For this review, take the finished solid that the model builds, in its own axes (mm). Give positions to 0.01 mm unless a question says otherwise; leave off trailing zeros. Loops run counter-clockwise (first coordinate to the right, second up) from the corner with the lowest first, then second, coordinate; pieces in that order, holes last.
```python
from build123d import *

# Parameters (mm, degrees)
ESQUISSE1_R             = 57.75
BOSS_EXTRU_1_DEPTH      = 1
ESQUISSE2_R             = 4
ENL_V_MAT_EXTRU_1_DEPTH = 10
ENL_V_MAT_EXTRU_4_DEPTH = 10
ESQUISSE5_R             = 1.5
ENL_V_MAT_EXTRU_5_DEPTH = 10


with BuildPart() as part:
    # Esquisse1 → Boss.-Extru.1 (new body)
    with BuildSketch(Plane.XY):
        Circle(ESQUISSE1_R)
    extrude(amount=BOSS_EXTRU_1_DEPTH)

    # Esquisse2 → Enlèv. mat.-Extru.1 (cut)
    with BuildSketch(Plane.XY.offset(1)):
        Circle(ESQUISSE2_R)
    extrude(amount=-ENL_V_MAT_EXTRU_1_DEPTH, mode=Mode.SUBTRACT)

    # Esquisse4 → Enlèv. mat.-Extru.4 (cut)
    with BuildSketch(Plane(origin=(0, 0, 0), x_dir=(-1, 0, 0), z_dir=(0, 0, -1))):
        with BuildLine():
            Line((33.243703386, 10.947884963), (53.229228234, 18.16877802))
            ThreePointArc((53.229228234, 18.16877802), (55.31077904, 10.615789501), (56.184630477, 2.830105651))
            Line((56.184630477, 2.830105651), (34.934630477, 2.138128484))
            ThreePointArc((34.934630477, 2.138128484), (34.372579979, 6.597404459), (33.243703386, 10.947884963))
        make_face()
    extrude(amount=-ENL_V_MAT_EXTRU_4_DEPTH, mode=Mode.SUBTRACT)

    # Esquisse5 → Enlèv. mat.-Extru.5 (cut)
    with BuildSketch(Plane(origin=(0, 0, 0), x_dir=(-1, 0, 0), z_dir=(0, 0, -1))):
        with Locations((0.504599234, -15.495791231)):
            Circle(ESQUISSE5_R)
    extrude(amount=-ENL_V_MAT_EXTRU_5_DEPTH, mode=Mode.SUBTRACT)


solid = part.part
```
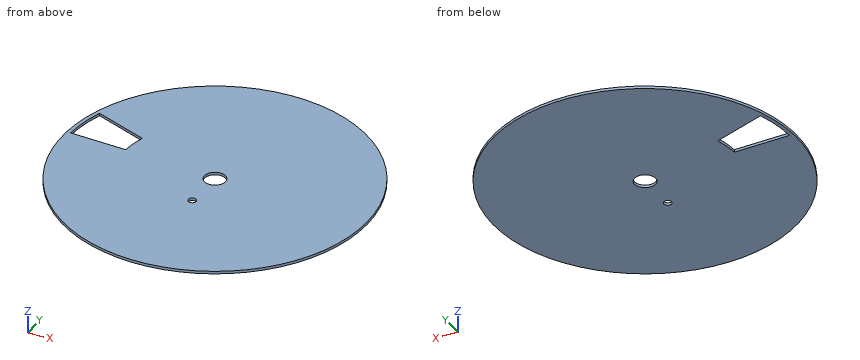
Q1. For probe 1 along Y at (x, z) = (0, 0.4); probe 2 along X at (y, z) = (7, 0.1); probe 3 along Y at (x, z) = (2.5, 0.4), list the stretches that pass through material, from the lowest coordinate up.
Answers:
probe 1: y = -57.75 to -16.91, -14.08 to -4, 4 to 57.75
probe 2: x = -57.32 to -55.87, -34.29 to 57.32
probe 3: y = -57.7 to -3.12, 3.12 to 57.7
Q2. Consider section A-A on y = 0. Give the boundary of the cut face in (x, z), plus the area to 4 significant figures.
Answers:
outline: (-57.75, 0) - (-4, 0) - (-4, 1) - (-57.75, 1) - close; (4, 0) - (57.75, 0) - (57.75, 1) - (4, 1) - close
area: 107.5 mm2
Q3. Consider section C-C on y = 30.5. Give the boundary of the cut face in (x, z).
Answers:
outline: (-49.04, 0) - (49.04, 0) - (49.04, 1) - (-49.04, 1) - close
Q4. Consider section B-B on z = 0.7. Give the boundary of the cut face in (x, y), plus the area to 3 significant figures.
Answers:
outline: circle Ø115.5 at (0, 0); hole (-56.18, 2.83) - (-34.93, 2.14) arc R35 cw to (-33.24, 10.95) - (-53.23, 18.17) arc R49.91 ccw to start; hole circle Ø8 at (0, 0); hole circle Ø3 at (-0.5, -15.5)
area: 10,200 mm2
